Here's how the part is built. I have some questions about the finished solid (model axes, mm). A direction names the side the tool comes from. Coordinates: 2 decimals unless noted, no trailing zeros. Write each loop counter-clockwise with the first axis right and the second up, starting at its lowest first coordinate (ties: lowest second). Pieces come first, ordered by that corner, then holes.
Item 1: For faces 4 (the face through (-6, 18, -3.2)), 5 (the face through (-9.44, 1.62, -29.03)), which set-ups out of +Z, -Z, +X, -X, +Y, -Y let a thin tool reach every point of the face, with its end or its side?
Item 2: I'm going to push flat-ended pins straight in: P1, Ø13, axis at x = 2.5, y = 25.5, coming from the -Z side; P2, Ø5, axis at x = 10, z = -7.5, coming from the +Y side; P3, Ø3.5, axis at x = 8.5, z = -19.5, coming from the -Y side. Where does each tip first touch, or does it pass through?
Item 3: Please list where these lines run through material, in increasing order: line 1 (X direction, y = 2.95, z = -19.5); line 2 (X direction, y = 25.5, z = -0.65); line 3 (X direction, y = 1, z = -19).
Item 4: If we mould it in two halves opening along X, with no side actions, what happens to faces 1 (the face through (0, 0, -14)), 2 (the face through (-1.46, 1.58, -23.01)), 3 (the face through (13.2, 10, -3))? For each: pulls with the +X half, pulls with the -X half, needs draft (parallel to the pull), parting line crosses it, or undercut.
Item 5: I want a section at C-C (y = 26). Please give me the cut outline in (x, z), and give its area (3 significant figures).
Item 6: I want a section at B-B (x = -1.5). Please give me the cut outline in (y, z).
Item 7: I want a section at D-D (x = 8.5). Please give me the cut outline in (y, z), and give its area (3 significant figures).
Item 8: I want a section at A-A (x = -4.25). Please give me the cut outline in (y, z), and give its area (3 significant figures).
from build123d import *

# Parameters (mm, degrees)
PAD_DEPTH       = 13.2
SKETCH001_R     = 3.8
SKETCH001_R_2   = 1.5
POCKET_DEPTH    = 33.001
SKETCH002_R     = 4.8
SKETCH002_R_2   = 1.65
POCKET001_DEPTH = 33.001
CHAMFER_SIZE    = 2
FILLET_R        = 13.19


with BuildPart() as part:
    # Sketch → Pad (new body, symmetric)
    with BuildSketch(Plane.YZ):
        with BuildLine():
            Line((33, 0), (3, 0))
            ThreePointArc((3, 0), (0.87868, -0.87868), (0, -3))
            Line((0, -3), (0, -33))
            Line((0, -33), (3.2, -33))
            Line((3.2, -33), (3.2, -4.2))
            ThreePointArc((4.2, -3.2), (3.492893, -3.492893), (3.2, -4.2))
            Line((4.2, -3.2), (33, -3.2))
            Line((33, -3.2), (33, 0))
        make_face()
    extrude(amount=PAD_DEPTH, both=True)

    # Sketch001 (on Face5 of Pad) → Pocket (cut, through all)
    with BuildSketch(Plane(origin=(0, 0, 0), x_dir=(0, 0, -1), z_dir=(0, -1, 0))):
        with Locations((19.5, 0)):
            Circle(SKETCH001_R)
        with Locations((19.5, 8.5)):
            Circle(SKETCH001_R_2)
        with Locations((19.5, -8.5)):
            Circle(SKETCH001_R_2)
    extrude(amount=-POCKET_DEPTH, mode=Mode.SUBTRACT)

    # Sketch002 (on Face7 of Pocket) → Pocket001 (cut, through all)
    with BuildSketch(Plane(origin=(0, 0, 0), x_dir=(0, -1, 0), z_dir=(0, 0, 1))):
        with Locations((-18.5, 0)):
            Circle(SKETCH002_R)
        with Locations((-11.5, 8)):
            Circle(SKETCH002_R_2)
        with Locations((-25.5, 8)):
            Circle(SKETCH002_R_2)
        with Locations((-25.5, -8)):
            Circle(SKETCH002_R_2)
        with Locations((-11.5, -8)):
            Circle(SKETCH002_R_2)
    extrude(amount=-POCKET001_DEPTH, mode=Mode.SUBTRACT)

    # Chamfer
    chamfer_edges = [part.edges().sort_by_distance(p)[0] for p in [
        (-8.5, 0, -18),
        (8.5, 0, -18),
    ]]
    chamfer(chamfer_edges, length=CHAMFER_SIZE)

    # Fillet
    fillet_edges = [part.edges().sort_by_distance(p)[0] for p in [
        (-13.2, 1.6, -33),
        (13.2, 1.6, -33),
    ]]
    fillet(fillet_edges, radius=FILLET_R)


solid = part.part
Answer:
1. face 4: -Z, +X, -X, +Y
1. face 5: -Z, -X, +Y, -Y
2. P1: stops at z = -3.2
2. P2: stops at y = 3.2
2. P3: stops at y = 1.75
3. line 1: x = -13.2 to -10, -7 to -3.8, 3.8 to 7, 10 to 13.2
3. line 2: x = -13.2 to -9.65, -6.35 to 6.35, 9.65 to 13.2
3. line 3: x = -13.2 to -10.95, -6.05 to -3.77, 3.77 to 6.05, 10.95 to 13.2
4. face 1: needs draft
4. face 2: undercut
4. face 3: pulls with the +X half
5. outline: (-13.2, -3.2) - (-9.57, -3.2) - (-9.57, 0) - (-13.2, 0) - close; (-6.43, -3.2) - (6.43, -3.2) - (6.43, 0) - (-6.43, 0) - close; (9.57, -3.2) - (13.2, -3.2) - (13.2, 0) - (9.57, 0) - close
5. area: 64.4 mm2
6. outline: (0, -32.92) - (3.2, -32.92) - (3.2, -22.99) - (0, -22.99) - close; (0, -16.01) - (3.2, -16.01) - (3.2, -4.2) arc R1 cw to (4.2, -3.2) - (13.94, -3.2) - (13.94, 0) - (3, 0) arc R3 ccw to (0, -3) - close; (23.06, -3.2) - (33, -3.2) - (33, 0) - (23.06, 0) - close
7. outline: (0, -29.9) - (3.2, -29.9) - (3.2, -21) - (2, -21) - (0, -23) - close; (0, -16) - (2, -18) - (3.2, -18) - (3.2, -4.2) arc R1 cw to (4.2, -3.2) - (9.93, -3.2) - (9.93, 0) - (3, 0) arc R3 ccw to (0, -3) - close; (13.07, -3.2) - (23.93, -3.2) - (23.93, 0) - (13.07, 0) - close; (27.07, -3.2) - (33, -3.2) - (33, 0) - (27.07, 0) - close
7. area: 156 mm2
8. outline: (0, -32.3) - (3.2, -32.3) - (3.2, -4.2) arc R1 cw to (4.2, -3.2) - (16.27, -3.2) - (16.27, 0) - (3, 0) arc R3 ccw to (0, -3) - close; (20.73, -3.2) - (33, -3.2) - (33, 0) - (20.73, 0) - close
8. area: 183 mm2
